Here's how the part is built. I have some questions about the finished solid (model axes, mm). A direction names the side the tool comes from. Give positions to 0.01 mm unless a question says otherwise; leave off trailing zeros. Order: outer loops, then holes, each group sorted by start corner. A loop starts at its lowest first (then second) coordinate and runs counter-clockwise, first axis right, second up. Notation, with made-up numbers: M -3,-25.75 L 38,-25.75 A22 ccw 38,-6.75 Z; hole C -15.5,8.5 d10. An arc over 180 degrees is marked long. Use one line per item in the form item = value.
from build123d import *

# Parameters (mm, degrees)
SKETCH1_R           = 2
SKETCH1_R_2         = 5
SKETCH1_R_3         = 10.5
SKETCH1_R_4         = 2.25
BOSS_EXTRUDE1_DEPTH = 3
SKETCH2_R           = 5
BOSS_EXTRUDE2_DEPTH = 3
CHAMFER2_SIZE       = 20
CHAMFER3_SIZE       = 40
SKETCH3_R           = 2
CUT_EXTRUDE1_DEPTH  = 10
SKETCH5_R           = 2.25
CUT_EXTRUDE2_DEPTH  = 10
SKETCH6_R           = 2
CUT_EXTRUDE3_DEPTH  = 171
SKETCH7_R           = 2
CUT_EXTRUDE4_DEPTH  = 22


with BuildPart() as part:
    # Sketch1 → Boss-Extrude1 (new body)
    with BuildSketch(Plane(origin=(0, 0, 0), x_dir=(1, 0, 0), z_dir=(0, 1, 0))):
        with BuildLine():
            Line((-200.2851606, -142.500000035), (-280, -142.500000035))
            ThreePointArc((-280, -142.500000035), (-294.999999965, -157.5), (-280, -172.499999965))
            Line((-280, -172.499999965), (280, -172.499999965))
            ThreePointArc((280, -172.499999965), (294.999999965, -157.5), (280, -142.500000035))
            Line((280, -142.500000035), (199.7148394, -142.500000035))
            Line((199.7148394, -142.500000035), (199.7148394, 187.499999965))
            Line((199.7148394, 187.499999965), (-160.2851606, 187.499999965))
            Line((-160.2851606, 187.499999965), (-160.2851606, 217.499999965))
            ThreePointArc((-160.2851606, 217.499999965), (-180.2851606, 237.499999965), (-200.2851606, 217.499999965))
            Line((-200.2851606, 217.499999965), (-200.2851606, 187.499999965))
            Line((-200.2851606, 187.499999965), (-200.2851606, -142.500000035))
        make_face()
        with Locations(Location((-157.5, 157.5, 0), (0, 0, 270))):
            Circle(SKETCH1_R, mode=Mode.SUBTRACT)
        with Locations(Location((157.5, 157.5, 0), (0, 0, 270))):
            Circle(SKETCH1_R, mode=Mode.SUBTRACT)
        with Locations(Location((157.5, -157.5, 0), (0, 0, 270))):
            Circle(SKETCH1_R, mode=Mode.SUBTRACT)
        with Locations(Location((-157.5, -157.5, 0), (0, 0, 270))):
            Circle(SKETCH1_R, mode=Mode.SUBTRACT)
        with Locations(Location((-280, -157.5, 0), (0, 0, 270))):
            Circle(SKETCH1_R_2, mode=Mode.SUBTRACT)
        with Locations(Location((280, -157.5, 0), (0, 0, 270))):
            Circle(SKETCH1_R_2, mode=Mode.SUBTRACT)
        with Locations(Location((-250, -157.5, 0), (0, 0, 270))):
            Circle(SKETCH1_R, mode=Mode.SUBTRACT)
        with Locations(Location((250, -157.5, 0), (0, 0, 270))):
            Circle(SKETCH1_R, mode=Mode.SUBTRACT)
        with Locations(Location((-180.2851606, 7.499999983, 0), (0, 0, 270))):
            Circle(SKETCH1_R_3, mode=Mode.SUBTRACT)
        with Locations(Location((-180.2851606, 20.999999983, 0), (0, 0, 270))):
            Circle(SKETCH1_R_4, mode=Mode.SUBTRACT)
        with Locations(Location((-180.2851606, -6.000000017, 0), (0, 0, 270))):
            Circle(SKETCH1_R_4, mode=Mode.SUBTRACT)
        with Locations(Location((180.2851606, -6.000000017, 0), (0, 0, 90))):
            Circle(SKETCH1_R_4, mode=Mode.SUBTRACT)
        with Locations(Location((180.2851606, 20.999999983, 0), (0, 0, 90))):
            Circle(SKETCH1_R_4, mode=Mode.SUBTRACT)
        with Locations(Location((180.2851606, 7.499999983, 0), (0, 0, 90))):
            Circle(SKETCH1_R_3, mode=Mode.SUBTRACT)
        with Locations(Location((-180.2851606, 217.499999965, 0), (0, 0, 270))):
            Circle(SKETCH1_R_2, mode=Mode.SUBTRACT)
    extrude(amount=BOSS_EXTRUDE1_DEPTH)

    # Sketch2 → Boss-Extrude2 (add)
    with BuildSketch(Plane(origin=(0, 3, 0), x_dir=(1, 0, 0), z_dir=(0, 1, 0))):
        with BuildLine():
            Line((199.7148394, 187.499999965), (199.7148394, 217.499999965))
            ThreePointArc((199.7148394, 217.499999965), (179.7148394, 237.499999965), (159.7148394, 217.499999965))
            Line((159.7148394, 217.499999965), (159.7148394, 187.499999965))
            Line((159.7148394, 187.499999965), (199.7148394, 187.499999965))
        make_face()
        with Locations(Location((179.7148394, 217.499999965, 0), (0, 0, 270))):
            Circle(SKETCH2_R, mode=Mode.SUBTRACT)
    extrude(amount=-BOSS_EXTRUDE2_DEPTH)

    # Chamfer2
    chamfer2_edges = [part.edges().sort_by_distance(p)[0] for p in [
        (-160.2851606, 1.5, -187.499999965),
        (159.7148394, 1.5, -187.499999965),
    ]]
    chamfer(chamfer2_edges, length=CHAMFER2_SIZE)

    # Chamfer3
    chamfer3_edges = [part.edges().sort_by_distance(p)[0] for p in [
        (-200.2851606, 1.5, 142.500000035),
        (199.7148394, 1.5, 142.500000035),
    ]]
    chamfer(chamfer3_edges, length=CHAMFER3_SIZE)

    # Sketch3 → Cut-Extrude1 (cut)
    with BuildSketch(Plane(origin=(0, 3, 0), x_dir=(1, 0, 0), z_dir=(0, 1, 0))):
        with Locations(Location((-180.2851606, 187.499999965, 0), (0, 0, 270))):
            Circle(SKETCH3_R)
    cut_extrude1 = extrude(amount=-CUT_EXTRUDE1_DEPTH, mode=Mode.SUBTRACT)

    # Mirror1: Cut-Extrude1 across plane
    add(cut_extrude1.mirror(Plane(origin=(0, 0, 0), x_dir=(0, 0, 1), z_dir=(1, 0, 0))), mode=Mode.SUBTRACT)

    # Sketch5 → Cut-Extrude2 (cut)
    with BuildSketch(Plane(origin=(0, 3, 0), x_dir=(1, 0, 0), z_dir=(0, 1, 0))):
        with Locations(Location((118.125, -118.125, 0), (0, 0, 270))):
            Circle(SKETCH5_R)
        with Locations(Location((78.75, -78.75, 0), (0, 0, 270))):
            Circle(SKETCH5_R)
        with Locations(Location((39.375, -39.375, 0), (0, 0, 270))):
            Circle(SKETCH5_R)
        with Locations(Location((-39.375, -39.375, 0), (0, 0, 270))):
            Circle(SKETCH5_R)
        with Locations(Location((-78.75, -78.75, 0), (0, 0, 270))):
            Circle(SKETCH5_R)
        with Locations(Location((-118.125, -118.125, 0), (0, 0, 270))):
            Circle(SKETCH5_R)
        with Locations(Location((-39.375, 39.375, 0), (0, 0, 270))):
            Circle(SKETCH5_R)
        with Locations(Location((-78.75, 78.75, 0), (0, 0, 270))):
            Circle(SKETCH5_R)
        with Locations(Location((-118.125, 118.125, 0), (0, 0, 270))):
            Circle(SKETCH5_R)
        with Locations(Location((39.375, 39.375, 0), (0, 0, 270))):
            Circle(SKETCH5_R)
        with Locations(Location((78.75, 78.75, 0), (0, 0, 270))):
            Circle(SKETCH5_R)
        with Locations(Location((118.125, 118.125, 0), (0, 0, 270))):
            Circle(SKETCH5_R)
        with Locations(Location((0, 0, 0), (0, 0, 270))):
            Circle(SKETCH5_R)
    extrude(amount=-CUT_EXTRUDE2_DEPTH, mode=Mode.SUBTRACT)

    # Sketch6 → Cut-Extrude3 (cut)
    with BuildSketch(Plane(origin=(0, 3, 0), x_dir=(1, 0, 0), z_dir=(0, 1, 0))):
        with Locations(Location((0, 157.5, 0), (0, 0, 270))):
            Circle(SKETCH6_R)
        with Locations(Location((-187.5, -157.5, 0), (0, 0, 270))):
            Circle(SKETCH6_R)
        with Locations(Location((187.5, -157.5, 0), (0, 0, 270))):
            Circle(SKETCH6_R)
    extrude(amount=-CUT_EXTRUDE3_DEPTH, mode=Mode.SUBTRACT)

    # Sketch7 → Cut-Extrude4 (cut)
    with BuildSketch(Plane(origin=(0, 3, 0), x_dir=(1, 0, 0), z_dir=(0, 1, 0))):
        with Locations(Location((0, 172.5, 0), (0, 0, 270))):
            Circle(SKETCH7_R)
    extrude(amount=-CUT_EXTRUDE4_DEPTH, mode=Mode.SUBTRACT)


solid = part.part
Q1. I want a section at C-C on z = -49.5. Write out the boundary of the cut face in (x, y), then the cut area to 3 significant figures.
Found:
outline = M -200.29,0 L 199.71,0 L 199.71,3 L -200.29,3 Z
area = 1,200 mm²
Q2. I want a section at B-B on x = -69. Write out the boundary of the cut face in (y, z), then the cut area to 3 significant figures.
Found:
outline = M 0,-187.5 L 3,-187.5 L 3,172.5 L 0,172.5 Z
area = 1,080 mm²
Q3. I'm going to push a flat-ended pin straight in: pin 1 Ø1 at (y, z) = (2, 13.5) entering from -X. Where does the tip first touch, or does it pass through?
Found:
pin_1 = -200.29
Q4. On a 3-axis mill with a long thin cutter (end or side, diameter ignored), from which of +Z, -Z, +X, -X, +Y, -Y can I reach the whole of each face in a straight line? I mean faces 1 (the face through (-169.875, 1.479, -8.867)), 2 (the face through (-150.145, 1.479, -197.36)). Say none if no direction works.
Found:
face_1 = +Y, -Y
face_2 = -Z, +Y, -Y
Q5. I need wall thicknesses on L1, parallel to X at y = 1.95, z = 6; L2, parallel to Z at x = 1, y = 0.15; L3, parallel to X at y = 0.85, z = 0. Which ranges of each line are inside material? Lowest first, please.
Found:
L1 = -200.29 to -182.54, -178.04 to 178.04, 182.54 to 199.71
L2 = -187.5 to -174.23, -170.77 to -159.23, -155.77 to -2.02, 2.02 to 172.5
L3 = -200.29 to -187.63, -172.94 to -2.25, 2.25 to 172.94, 187.63 to 199.71
Q6. Thinking about a two-plate mould opening in X: for faces 3 (the face through (219.995, 1.479, 122.78)), 4 (the face through (-294.996, 1.479, 157.17)), 5 (the face through (149.855, 1.521, -197.64)), which applies, +X half, -X half, draft (parallel to the pull), parting line (faces both ways), or undercut?
Found:
face_3 = +X half
face_4 = -X half
face_5 = undercut
Q7. I want a section at A-A on y = 1.75. State how many separate pieces and enclosed holes the cut face has, then the cut area to 3 significant figures.
Found:
separate_pieces = 1
enclosed_holes = 35
area = 154,000 mm²
